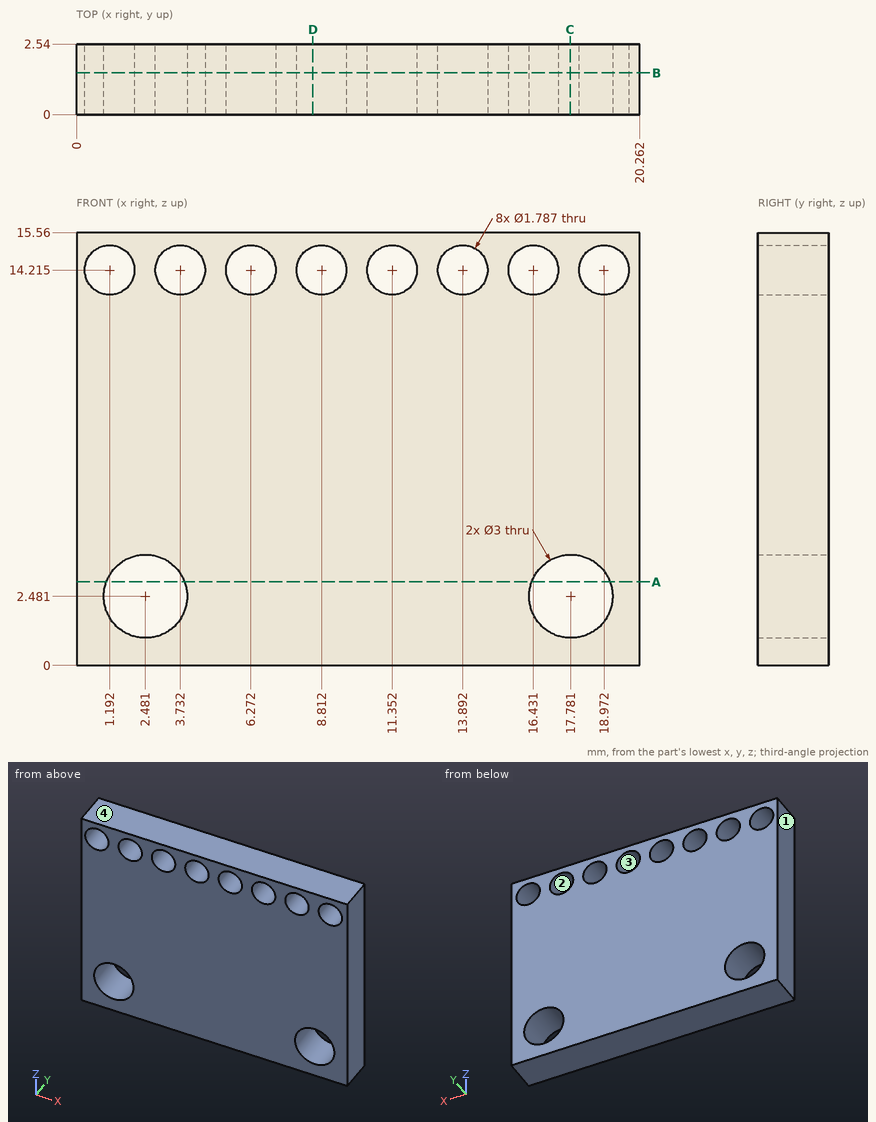
Design review of the part shown in the three views and the two pictorial views. Dimensions are in mm from the part's minimum x, y and z. Give positions to 0.01 mm unless a question says otherwise; leave off trailing zeros. Write each loop counter-clockwise with the first axis right and the second up, starting at its lowest first coordinate (ties: lowest second). Pieces come first, ordered by that corner, then holes. Notation, with made-up numbers: M 88,34 L 98,34 A25 cw 98,59 Z; hole C 30,8 d11. An arc over 180 degrees is marked long. One line per question, with ' | ' between items. Start each with the question number.
Item 1: We need section D-D on x = 8.5. Write out the cut boundary in (y, z).
Item 2: We need section A-A on z = 3. Write out the cut boundary in (x, y).
Item 3: We need section C-C on x = 17.75. Write out the cut boundary in (y, z), plus the area to 3 significant figures.
Item 4: Draft analysis for pull direction X (two halves, no side actions). For the marked faces 1, 2, 3 and 4, state which applies: released by +X, released by -X, zero draft, split by the parting line, or undercut.
Item 5: Wall thickness on line 1 (Z direction, x = 8.75, y = 2); line 2 (X direction, y = 2.15, z = 2.75) (1 decimal); line 3 (X direction, y = 2.25, z = 3) (1 decimal): over which ranges is each line inside the solid? List them lowest first. Write a range as from..to.
Item 6: For pin 1 (1.6 mm diameter, centred on x = 3.73, z = 14.22, fed in from +Y), flat-tipped, find the tip position at first contact; note if it passes through.
Item 7: We need section B-B on y = 1.5. Give the number of separate pieces and of enclosed holes in the cut face, plus the area to 3 significant figures.
Results found:
1) outline: M 0,0 L 2.54,0 L 2.54,13.38 L 0,13.38 Z; M 0,15.05 L 2.54,15.05 L 2.54,15.56 L 0,15.56 Z
2) outline: M 0,0 L 1.07,0 L 1.07,2.54 L 0,2.54 Z; M 3.89,0 L 16.37,0 L 16.37,2.54 L 3.89,2.54 Z; M 19.19,0 L 20.26,0 L 20.26,2.54 L 19.19,2.54 Z
3) outline: M 0,0 L 2.54,0 L 2.54,0.98 L 0,0.98 Z; M 0,3.98 L 2.54,3.98 L 2.54,15.56 L 0,15.56 Z | area: 31.9 mm2
4) face 1: released by -X | face 2: undercut | face 3: undercut | face 4: zero draft
5) line 1: z = 0..13.32, 15.11..15.56 | line 2: x = 0..1, 4..16.3, 19.3..20.3 | line 3: x = 0..1.1, 3.9..16.4, 19.2..20.3
6) pin 1: passes through
7) separate pieces: 1 | enclosed holes: 10 | area: 281 mm2
